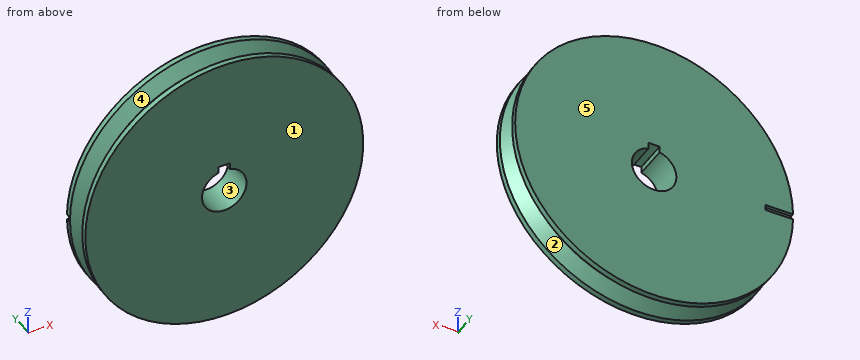
```python
from build123d import *

# Parameters (mm, degrees)
CUT_EXTRUDE1_DEPTH = 180.30421077
CUT_EXTRUDE3_START = -3
CUT_EXTRUDE3_DEPTH = 3


with BuildPart() as part:
    # Sketch1 → Revolve1 (revolve)
    with BuildSketch(Plane.XY, mode=Mode.PRIVATE) as revolve1_sk:
        Polygon((0, 15), (125, 15), (125, 10), (115, 0), (125, -10), (125, -15), (0, -15), align=None)
    revolve(revolve1_sk.sketch.rotate(Axis((0, -15, 0), (0, -1, 0)), 180), axis=Axis((0, -15, 0), (0, -1, 0)))

    # Sketch2 → Cut-Extrude1 (cut, through all)
    with BuildSketch(Plane(origin=(0, 15, 0), x_dir=(-1, 0, 0), z_dir=(0, 1, 0))):
        with BuildLine():
            Line((-5, 19.364916731), (-5, 25))
            Line((-5, 25), (5, 25))
            Line((5, 25), (5, 19.364916731))
            ThreePointArc((5, 19.364916731), (0, -20), (-5, 19.364916731))
        make_face()
    extrude(amount=-CUT_EXTRUDE1_DEPTH, mode=Mode.SUBTRACT)

    # Sketch3 → Cut-Extrude3 (cut)
    with BuildSketch(Plane(origin=(0, 15, 0), x_dir=(-1, 0, 0), z_dir=(0, 1, 0)).offset(CUT_EXTRUDE3_START)):
        with BuildLine():
            Line((99.974997499, -2.5), (124.974997499, -2.5))
            ThreePointArc((124.974997499, -2.5), (125, 0), (124.974997499, 2.5))
            Line((124.974997499, 2.5), (99.974997499, 2.5))
            Line((99.974997499, 2.5), (99.974997499, -2.5))
        make_face()
    extrude(amount=CUT_EXTRUDE3_DEPTH, mode=Mode.SUBTRACT)


solid = part.part
```
Source: CAD feature listing. Evaluate the final solid. Frame: model axes, mm. Face numbers are marked on the shaded views. A direction names the side the tool comes from. Give positions to 0.01 mm unless a question says otherwise; leave off trailing zeros. Write each loop counter-clockwise with the first axis right and the second up, starting at its lowest first coordinate (ties: lowest second). Pieces come first, ordered by that corner, then holes.
1. Access query for the marked faces 1 and 2. Directions: +Z, -Z, +X, -X, +Y, -Y. A direction counts if a zero-diameter tool reaches every point of the face in a straight line with its end or side. Return the directions, or none.
2. Material intervals for line 1 along Z through (x, y) = (0, 8.25); line 2 along Z through (x, y) = (16, -11.5); line 3 along Y through (x, z) = (61, 100), sorted ascending.
3. Pull-direction query (X, two-part tool) for the marked faces 3, 4 and 5; classes: +X half, -X half, draft (parallel to the pull), parting line (faces both ways), or undercut.
4. First-contact query: pin 1 (3.5 mm diameter, centred on x = -107.5, y = 14, fed in from -Z); pin 2 (8 mm diameter, centred on x = 86.5, y = -8.5, fed in from +Z); pin 3 (11 mm diameter, centred on x = -1, y = 3, fed in from -Z). Flat tips, straight axial feed; report the tip coordinate or a pass-through.
5. Section query A-A (x = 0). Return the cut outline in (y, z).
Output values:
1. face 1: +Z, -Z, +X, -X, -Y
1. face 2: none
2. line 1: z = -123.25 to -20, 25 to 123.25
2. line 2: z = -123.97 to -12, 12 to 123.97
2. line 3: y = -15 to -2.14, 2.14 to 15
3. face 3: undercut
3. face 4: parting line
3. face 5: draft
4. pin 1: stops at z = -66.65
4. pin 2: stops at z = 93.65
4. pin 3: stops at z = -123.5
5. outline: (-15, -125) - (-10, -125) - (0, -115) - (10, -125) - (15, -125) - (15, -20) - (-15, -20) - close; (-15, 25) - (15, 25) - (15, 125) - (10, 125) - (0, 115) - (-10, 125) - (-15, 125) - close
